Model file for the job. Use its own axes, mm. Give positions to 0.01 mm unless a question says otherwise; leave off trailing zeros. Loops run counter-clockwise (first coordinate to the right, second up) from the corner with the lowest first, then second, coordinate; pieces in that order, holes last. Notation, with made-up numbers: M 32.25,88 L 84.25,88 A14 ccw 84.25,104 Z; hole C 0,10.25 d3. An arc over 180 degrees is marked long. Answer in a Markdown table with one row per item.
```python
from build123d import *

# Parameters (mm, degrees)
SKETCH1_R           = 150
SKETCH1_W           = 59.5
SKETCH1_H           = 84.9
BOSS_EXTRUDE1_DEPTH = 3
SKETCH3_R           = 1.4224
SKETCH3_R_2         = 3.175
SKETCH3_W           = 3
SKETCH3_H           = 3
CUT_EXTRUDE1_DEPTH  = 10
SKETCH6_W           = 80
SKETCH6_H           = 88.399519522
CUT_EXTRUDE3_DEPTH  = 3
SKETCH8_R           = 1.4224
CUT_EXTRUDE5_DEPTH  = 3


with BuildPart() as part:
    # Sketch1 → Boss-Extrude1 (new body)
    with BuildSketch(Plane(origin=(0, 0, 0), x_dir=(1, 0, 0), z_dir=(0, 1, 0))):
        Circle(SKETCH1_R)
        Rectangle(SKETCH1_W, SKETCH1_H, mode=Mode.SUBTRACT)
    extrude(amount=BOSS_EXTRUDE1_DEPTH)

    # Sketch3 → Cut-Extrude1 (cut)
    with BuildSketch(Plane(origin=(0, 3, 0), x_dir=(1, 0, 0), z_dir=(0, 1, 0))):
        with Locations((-40.9, 45.7)):
            Circle(SKETCH3_R)
        with Locations((40.9, 45.7)):
            Circle(SKETCH3_R)
        with Locations((40.9, -45.7)):
            Circle(SKETCH3_R)
        with Locations((-40.9, -45.7)):
            Circle(SKETCH3_R)
        with Locations((-102.7, 27.7)):
            Circle(SKETCH3_R_2)
        with Locations((-102.7, -27.7)):
            Circle(SKETCH3_R_2)
        with Locations((102.7, 27.7)):
            Circle(SKETCH3_R_2)
        with Locations((102.7, -27.7)):
            Circle(SKETCH3_R_2)
        with Locations((-48.5, 45.7)):
            Rectangle(SKETCH3_W, SKETCH3_H)
        with Locations((48.5, 45.7)):
            Rectangle(SKETCH3_W, SKETCH3_H)
        with Locations((48.5, -45.7)):
            Rectangle(SKETCH3_W, SKETCH3_H)
        with Locations((-48.5, -45.7)):
            Rectangle(SKETCH3_W, SKETCH3_H)
    extrude(amount=-CUT_EXTRUDE1_DEPTH, mode=Mode.SUBTRACT)

    # Sketch6 → Cut-Extrude3 (cut)
    with BuildSketch(Plane(origin=(0, 3, 0), x_dir=(1, 0, 0), z_dir=(0, 1, 0))):
        with Locations((0, -117.129759761)):
            Rectangle(SKETCH6_W, SKETCH6_H)
    extrude(amount=-CUT_EXTRUDE3_DEPTH, mode=Mode.SUBTRACT)

    # Sketch8 → Cut-Extrude5 (cut)
    with BuildSketch(Plane.XZ):
        with Locations((100.762716319, 100.762716319)):
            Circle(SKETCH8_R)
        with Locations((93.691648507, 93.691648507)):
            Circle(SKETCH8_R)
        with Locations((100.762716319, -100.762716319)):
            Circle(SKETCH8_R)
        with Locations((93.691648507, -93.691648507)):
            Circle(SKETCH8_R)
        with Locations((-100.762716319, -100.762716319)):
            Circle(SKETCH8_R)
        with Locations((-93.691648507, -93.691648507)):
            Circle(SKETCH8_R)
        with Locations((-100.762716319, 100.762716319)):
            Circle(SKETCH8_R)
        with Locations((-93.691648507, 93.691648507)):
            Circle(SKETCH8_R)
        Polygon((90.633411679, 86.143283618), (92.754732022, 88.264603962), (88.264603962, 92.754732022), (86.143283618, 90.633411679), align=None)
        Polygon((103.820953148, 108.311081208), (108.311081208, 103.820953148), (106.189760865, 101.699632804), (101.699632804, 106.189760865), align=None)
        Polygon((86.143283618, -90.633411679), (88.264603962, -92.754732022), (92.754732022, -88.264603962), (90.633411679, -86.143283618), align=None)
        Polygon((108.311081208, -103.820953148), (103.820953148, -108.311081208), (101.699632804, -106.189760865), (106.189760865, -101.699632804), align=None)
        Polygon((-90.633411679, -86.143283618), (-92.754732022, -88.264603962), (-88.264603962, -92.754732022), (-86.143283618, -90.633411679), align=None)
        Polygon((-103.820953148, -108.311081208), (-108.311081208, -103.820953148), (-106.189760865, -101.699632804), (-101.699632804, -106.189760865), align=None)
        Polygon((-86.143283618, 90.633411679), (-88.264603962, 92.754732022), (-92.754732022, 88.264603962), (-90.633411679, 86.143283618), align=None)
        Polygon((-108.311081208, 103.820953148), (-103.820953148, 108.311081208), (-101.699632804, 106.189760865), (-106.189760865, 101.699632804), align=None)
    extrude(amount=-CUT_EXTRUDE5_DEPTH, mode=Mode.SUBTRACT)


solid = part.part
```
Q1. Saw through at C-C (y = 1.75). Give the number of separate pieces and of enclosed holes in the cut face, and give its area (3 significant figures).
Reported:
| item | result |
|---|---|
| separate pieces | 1 |
| enclosed holes | 25 |
| area | 59,200 mm² |
Q2. Probe probe 1 along Z at (x, y) = (-105, 0.1); probe 2 along X at (y, z) = (0.25, -99.5); probe 3 along X at (y, z) = (1.8, 27.5). List the from-to ranges inside material, lowest first.
Reported:
| item | result |
|---|---|
| probe 1 | -102.89 to -29.89, -25.51 to 25.51, 29.89 to 102.89 |
| probe 2 | -112.25 to -101.42, -100.11 to 100.11, 101.42 to 112.25 |
| probe 3 | -147.46 to -105.87, -99.53 to -29.75, 29.75 to 99.53, 105.87 to 147.46 |
Q3. Saw through at B-B (x = 20.5). Give the cut face in (y, z).
Reported:
| item | result |
|---|---|
| outline | M 0,-148.59 L 3,-148.59 L 3,-42.45 L 0,-42.45 Z; M 0,42.45 L 3,42.45 L 3,72.93 L 0,72.93 Z |
Q4. Drop flat-ended pins along their axis: pin 1 (8 mm diameter, centred on x = -109, z = 11, fed in from -Y); pin 2 (2.5 mm diameter, centred on x = -93.69, z = -93.69, fed in from -Y); pin 3 (1.5 mm diameter, centred on y = 2.5, z = -82.5, fed in from +X); pin 4 (1.5 mm diameter, centred on y = 1, z = -45.5, fed in from -X). Give the stop position or say it passes through.
Reported:
| item | result |
|---|---|
| pin 1 | y = 0 |
| pin 2 | through |
| pin 3 | x = 125.77 |
| pin 4 | x = -143.17 |
Q5. Saw through at A-A (z = -13.5). Give the cut face in (x, y), and give its area (3 significant figures).
Reported:
| item | result |
|---|---|
| outline | M -149.39,0 L -29.75,0 L -29.75,3 L -149.39,3 Z; M 29.75,0 L 149.39,0 L 149.39,3 L 29.75,3 Z |
| area | 718 mm² |
Q6. Mould opens along Z. For faces 1 (the face through (-105.22, 1.52, 29.63)), 2 (the face through (-149.99, 1.48, -1.6)), 3 (the face through (73.7, 1.479, 130.646)), 4 (the face through (31, 3, -5)) say: released by +Z, released by -Z, zero draft, split by the parting line, or undercut.
Reported:
| item | result |
|---|---|
| face 1 | undercut |
| face 2 | split by the parting line |
| face 3 | released by +Z |
| face 4 | zero draft |
Q7. Saw through at D-D (x = -125). Give the cut face in (y, z), and give its area (3 significant figures).
Reported:
| item | result |
|---|---|
| outline | M 0,-82.92 L 3,-82.92 L 3,82.92 L 0,82.92 Z |
| area | 497 mm² |
